Read the model definition and answer for the solid it produces. Units are mm, in the model's axes. A direction names the side the tool comes from. Coordinates: 2 decimals unless noted, no trailing zeros. Order: outer loops, then holes, each group sorted by start corner. A loop starts at its lowest first (then second) coordinate and runs counter-clockwise, first axis right, second up. Notation, with made-up numbers: (69.25, -16) - (122.25, -16) arc R30 cw to (122.25, 14) - close; hole circle Ø2 at (85.25, 16). An arc over 180 degrees is marked (long way). Use one line per item in the form item = value. Start each with the question number.
from build123d import *

# Parameters (mm, degrees)
SKETCH_1_R          = 18.75
SKETCH_1_R_2        = 14.5
EXTRUDE_1_DEPTH     = 16
SKETCH_2_R          = 1.25
CUT_EXTRUDE_1_DEPTH = 18
CUT_EXTRUDE_2_DEPTH = 18
SKETCH_4_R          = 18.75
EXTRUDE_2_DEPTH     = 2
SKETCH_6_R          = 1.25
EXTRUDE_3_DEPTH     = 16
SKETCH_7_R          = 1.25
CUT_EXTRUDE_3_DEPTH = 20


with BuildPart() as part:
    # 草图1 → 凸台-拉伸1 (new body)
    with BuildSketch(Plane.XY):
        Circle(SKETCH_1_R)
        Circle(SKETCH_1_R_2, mode=Mode.SUBTRACT)
    extrude(amount=EXTRUDE_1_DEPTH)

    # 草图2 → 切除-拉伸1 (cut)
    with BuildSketch(Plane.XY.offset(16)):
        with Locations((16.625, 0)):
            Circle(SKETCH_2_R)
        with Locations((-8.3125, -14.397672338)):
            Circle(SKETCH_2_R)
        with Locations((-8.3125, 14.397672338)):
            Circle(SKETCH_2_R)
    extrude(amount=-CUT_EXTRUDE_1_DEPTH, mode=Mode.SUBTRACT)

    # 草图3 → 切除-拉伸2 (cut)
    with BuildSketch(Plane.XY.offset(16)):
        with BuildLine():
            ThreePointArc((-7.142590701, -15.756693755), (8.65, -14.982239485), (17.216992422, -1.692681881))
            ThreePointArc((17.216992422, -1.692681881), (14.831783064, 0), (17.216992422, 1.692681881))
            ThreePointArc((17.216992422, 1.692681881), (8.65, 14.982239485), (-7.142590701, 15.756693755))
            ThreePointArc((-7.142590701, 15.756693755), (-7.415891532, 12.844700917), (-10.07440172, 14.064011873))
            ThreePointArc((-10.07440172, 14.064011873), (-17.3, 0), (-10.07440172, -14.064011873))
            ThreePointArc((-10.07440172, -14.064011873), (-7.415891532, -12.844700917), (-7.142590701, -15.756693755))
        make_face()
    extrude(amount=-CUT_EXTRUDE_2_DEPTH, mode=Mode.SUBTRACT)

    # 草图4 → 凸台-拉伸2 (add)
    with BuildSketch(Plane.XY.offset(16)):
        Circle(SKETCH_4_R)
    extrude(amount=EXTRUDE_2_DEPTH)

    # 草图6 → 凸台-拉伸3 (add)
    with BuildSketch(Plane(origin=(0, 0, 0), x_dir=(-1, 0, 0), z_dir=(0, 0, -1))):
        with Locations((8.3125, -14.397672338)):
            Circle(SKETCH_6_R)
        with Locations((-16.625, 0)):
            Circle(SKETCH_6_R)
        with Locations((8.3125, 14.397672338)):
            Circle(SKETCH_6_R)
    extrude(amount=-EXTRUDE_3_DEPTH)

    # 草图7 → 切除-拉伸3 (cut)
    with BuildSketch(Plane(origin=(0, 0, 0), x_dir=(-1, 0, 0), z_dir=(0, 0, -1))):
        with Locations((8.375, 14.505925513)):
            Circle(SKETCH_7_R)
        with Locations((8.375, -14.505925513)):
            Circle(SKETCH_7_R)
        with Locations((-16.75, 0)):
            Circle(SKETCH_7_R)
    extrude(amount=-CUT_EXTRUDE_3_DEPTH, mode=Mode.SUBTRACT)


solid = part.part
Q1. A cutting plane is placed at B-B (x = 16.75). Give the vertices of the cut face in (y, z), then the cut area to 3 significant figures.
Q2. For a pull along X with two mould halves and no side action, classify faces 1 (the flat face through (-7, -14, 0)), 2 (the cylindrical face through (-2.44, 18.59, 8.87)), 3 (the cylindrical face through (8.848, 14.866, 8.112)) as +X half, -X half, draft (parallel to the pull), parting line (faces both ways), or undercut.
Q3. Given P1, Ø1.5, axis at x = 12.5, y = -6, coming from the -Z side; P2, Ø10, axis at x = 7.5, z = 13, coming from the -Y side; P3, Ø5, axis at y = 14.5, z = 16, coming from the +X side; P4, Ø2, axis at x = 16.75, y = 0, coming from the +Z side, each flat-ended and moving along its own axis, determine where each tip first touches the part or whether it passes through.
Q4. A cutting plane is placed at C-C (z = 14.5). Give the number of separate pieces and of enclosed holes in the cut face, then the cut area to 3 significant figures.
Q5. Consider probe 1 along X at (y, z) = (13.5, 2.25); probe 2 along Y at (x, z) = (15, 14); probe 3 along X at (y, z) = (-15.5, 1.25). Determine where each line is inside the solid, lowest interval first.
Q6. A cutting plane is placed at D-D (x = -8.5). Give the vertices of the cut face in (y, z).
Q7. A cutting plane is placed at A-A (y = 0). Give the vertices of the cut face in (x, z).
Q8. Which of the six approach directions +Z, -Z, +X, -X, +Y, -Y give full straight-line access (tool end or side, diameter ignored) to faces 4 (the flat face through (0, 0, 16)), 5 (the cylindrical face through (-7.5, 15.4, 8.9))?
Result sheet:
q1.outline = (-8.43, 0) - (-4.33, 0) - (-4.33, 16) - (-1.79, 16) - (-1.79, 0) - (-1.25, 0) - (-1.25, 18) - (-8.43, 18) - close; (1.25, 0) - (1.79, 0) - (1.79, 16) - (4.33, 16) - (4.33, 0) - (8.43, 0) - (8.43, 18) - (1.25, 18) - close
q1.area = 177 mm^2
q2.face_1 = draft
q2.face_2 = parting line
q2.face_3 = undercut
q3.P1 = 16
q3.P2 = -18.58
q3.P3 = 14.41
q3.P4 = through
q4.separate_pieces = 1
q4.enclosed_holes = 4
q4.area = 171 mm^2
q5.probe_1 = -13.01 to -10.82, -9.86 to -9.12, -7.63 to -6.76, 10.82 to 13.01
q5.probe_2 = -11.25 to -8.62, -0.76 to 0.76, 8.62 to 11.25
q5.probe_3 = -10.55 to -9.13, -7.62 to -6.9, 7.68 to 10.55
q6.outline = (-16.71, 0) - (-15.75, 0) - (-15.75, 18) - (-16.71, 18) - close; (-13.26, 0) - (-12.61, 0) - (-12.61, 16) - (12.61, 16) - (12.61, 0) - (13.26, 0) - (13.26, 18) - (-13.26, 18) - close; (15.75, 0) - (16.71, 0) - (16.71, 18) - (15.75, 18) - close
q7.outline = (-18.75, 0) - (-17.3, 0) - (-17.3, 16) - (14.83, 16) - (14.83, 0) - (15.5, 0) - (15.5, 18) - (-18.75, 18) - close; (18, 0) - (18.75, 0) - (18.75, 18) - (18, 18) - close
q8.face_4 = -Z
q8.face_5 = +Z, -Z
